Here's how the part is built. I have some questions about the finished solid (model axes, mm). A direction names the side the tool comes from. Coordinates: 2 decimals unless noted, no trailing zeros.
```python
from build123d import *

# Parameters (mm, degrees)
BLANKSKE_W          = 500
BLANKSKE_H          = 24
BLANK_DEPTH         = 100
TOOTHCUTSIM_DEPTH   = 511.466453354
TEETHCUTS_COUNT     = 21
TEETHCUTS_PITCH     = 25.1327412
SKETCH1_W           = 800
SKETCH1_H           = 100
BOSS_EXTRUDE1_DEPTH = 30
SCALE1_SCALE        = 0.25
BOSS_EXTRUDE2_DEPTH = 7.5


with BuildPart() as part:
    # BlankSke → Blank (new body)
    with BuildSketch(Plane.XY):
        with Locations((250, 12)):
            Rectangle(BLANKSKE_W, BLANKSKE_H)
    extrude(amount=-BLANK_DEPTH)

    # TooCutSkeSim → ToothCutSim (cut, through all)
    with BuildSketch(Plane.XY):
        Polygon((3.408482957, 6), (-3.408482957, 6), (-9.969192018, 24.0254), (9.969192018, 24.0254), align=None)
    toothcutsim = extrude(amount=-TOOTHCUTSIM_DEPTH, mode=Mode.SUBTRACT)

    # TeethCuts: ToothCutSim ×21
    with Locations(*[(i * TEETHCUTS_PITCH, 0, 0) for i in range(1, TEETHCUTS_COUNT)]):
        add(toothcutsim, mode=Mode.SUBTRACT)

    # Sketch1 → Boss-Extrude1 (add)
    with BuildSketch(Plane.XZ):
        with Locations((99.246341043, -50)):
            Rectangle(SKETCH1_W, SKETCH1_H)
    extrude(amount=BOSS_EXTRUDE1_DEPTH)


with BuildPart() as part_1:
    # Scale1: scaled about (134.34613588, -9.4300262, -50)
    add(part.part.scale(SCALE1_SCALE).moved(Location((100.75960191, -7.07251965, -37.5))))

    # Sketch3 → Boss-Extrude2 (add)
    with BuildSketch(Plane(origin=(0, -7.07251965, 0), x_dir=(1, 0, 0), z_dir=(0, 1, 0))):
        with BuildLine():
            Line((96.237657296, 62.5), (25.57118717, 62.5))
            Line((25.57118717, 62.5), (25.57118717, 37.5))
            Line((25.57118717, 37.5), (96.237657296, 37.5))
            add(Edge.make_bspline(
                [(25.57118717, 0), (78.47502041, 0), (43.333824056, 37.5), (96.237657296, 37.5)],
                knots=[0, 0, 0, 0, 1, 1, 1, 1], degree=3))
            ThreePointArc((25.57118717, 0), (-24.42881283, 50), (25.57118717, 100))
            add(Edge.make_bspline(
                [(25.57118717, 100), (78.47502041, 100), (43.333824056, 62.5), (96.237657296, 62.5)],
                knots=[0, 0, 0, 0, 1, 1, 1, 1], degree=3))
        make_face()
    extrude(amount=-BOSS_EXTRUDE2_DEPTH)


solid = part_1.part
```
Q1. We'd pull the mould along X, two halves only. Please class faces 5 (the flat face through (224.764, -3.354, -49.825)), 6 (the flat face through (212.197, -3.354, -49.825)), 7 (the flat face through (160, -9, -62.5)): pulls with the +X half, pulls with the -X half, needs draft (parallel to the pull), parting line crosses it, or undercut.
Q2. For faces 1 (the flat face through (75, -14.573, -51)), 2 (the flat face through (225.571, -11, -50)), 3 (the flat face through (196.69, -3.29, -49.82)), 4 (the flat face through (160, -9, -37.5)), which set-ups out of +Z, -Z, +X, -X, +Y, -Y let a thin tool reach every point of the face, with its end or its side?
Q3. I need wall thicknesses on L1, parallel to Z at x = 186.5, y = -13; L2, parallel to Y at x = 81, z = -55.5; L3, parallel to Z at x = 74.5, y = -13.25. Which ranges of each line are inside material? Lowest first, please.
Q4. Will these pins go through, and if not, where does the flat tip stop? pin 1 (0.5 mm diameter, centred on x = 151, z = -54.5, fed in from +Y); pin 2 (7 mm diameter, centred on x = 171, y = -5, fed in from -Z); pin 3 (4 mm diameter, centred on x = 1, y = -7.5, fed in from -Z).
Reply:
1. face 5: pulls with the +X half
1. face 6: undercut
1. face 7: needs draft
2. face 1: +Z, -Z, +X, -X, -Y
2. face 2: +Z, -Z, +X, -Y
2. face 3: +Z, -Z, +Y
2. face 4: +Z, +X, +Y, -Y
3. L1: z = -62.5 to -37.5
3. L2: y = -14.57 to -7.07
3. L3: z = -66.01 to -33.99
4. pin 1: stops at y = -5.57
4. pin 2: stops at z = -62.5
4. pin 3: stops at z = -94.62
